from build123d import *

# Parameters (mm, degrees)
BOSS_EXTRUDE1_DEPTH = 20
SKETCH2_R           = 21
CUT_EXTRUDE1_DEPTH  = 21
SKETCH3_W           = 16
SKETCH3_H           = 76
BOSS_EXTRUDE2_DEPTH = 150


with BuildPart() as part:
    # Sketch1 → Boss-Extrude1 (new body)
    with BuildSketch(Plane.XY):
        with BuildLine():
            Line((0, 80), (0, 0))
            Line((0, 0), (60, 0))
            ThreePointArc((60, 0), (88.284271247, 11.715728753), (100, 40))
            ThreePointArc((100, 40), (88.284271247, 68.284271247), (60, 80))
            Line((60, 80), (0, 80))
        make_face()
    extrude(amount=BOSS_EXTRUDE1_DEPTH)

    # Sketch2 → Cut-Extrude1 (cut, through all)
    with BuildSketch(Plane.XY.offset(20)):
        with Locations((60, 40)):
            Circle(SKETCH2_R)
    extrude(amount=-CUT_EXTRUDE1_DEPTH, mode=Mode.SUBTRACT)

    # Sketch3 → Boss-Extrude2 (add)
    with BuildSketch(Plane.ZY):
        with Locations((10, 40)):
            Rectangle(SKETCH3_W, SKETCH3_H)
    extrude(amount=BOSS_EXTRUDE2_DEPTH)


solid = part.part
CAD build for the part. Positions are in the model's coordinates, mm. A direction names the side the tool comes from. Coordinates: 2 decimals unless noted, no trailing zeros. Order: outer loops, then holes, each group sorted by start corner. A loop starts at its lowest first (then second) coordinate and runs counter-clockwise, first axis right, second up. Notation, with made-up numbers: (29.25, -36) -> (86.25, -36) arc R18 cw to (86.25, -28) -> close; hole circle Ø1 at (-6.5, -12). An arc over 180 degrees is marked (long way). Answer in a Markdown table with one row per item.
1) Mould opens along Y. For faces 1 (the face through (38, 41, 0)), 2 (the face through (44.52, 54.19, 10.14)), 3 (the face through (-74, 2, 10)), 4 (the face through (-74, 78, 10)) say: pulls with the +Y half, pulls with the -Y half, needs draft (parallel to the pull), parting line crosses it, or undercut.
Check values:
| item | result |
|---|---|
| face 1 | needs draft |
| face 2 | undercut |
| face 3 | pulls with the -Y half |
| face 4 | pulls with the +Y half |
2) Which spindle directions (+Z, -Z, +X, -X, +Y, -Y) get a long thin tool onto all of the face, cutting with end or side? Do faces 5 (the face through (-150, 41, 10)), 6 (the face through (-74, 39, 2)), 7 (the face through (-74, 39, 18)). Say none if no direction does.
Check values:
| item | result |
|---|---|
| face 5 | +Z, -Z, -X, +Y, -Y |
| face 6 | -Z, -X, +Y, -Y |
| face 7 | +Z, -X, +Y, -Y |
3) Band-saw the part on D-D (x = -14.5). List the corners of the cut face in (y, z).
Check values:
| item | result |
|---|---|
| outline | (2, 2) -> (78, 2) -> (78, 18) -> (2, 18) -> close |
4) Band-saw the part on A-A (z = 5.5). List the corners of the cut face in (x, y), and give its area (3 significant figures).
Check values:
| item | result |
|---|---|
| outline | (-150, 2) -> (0, 2) -> (0, 0) -> (60, 0) arc R40 ccw to (60, 80) -> (0, 80) -> (0, 78) -> (-150, 78) -> close; hole circle Ø42 at (60, 40) |
| area | 17,300 mm2 |
5) Flat gauge pins, fed straight in: P1, Ø3, axis at x = -77.5, z = 6, coming from the +Y side; P2, Ø8, axis at y = 16, z = 7, coming from the +X side; P3, Ø23, axis at x = -92.5, y = 53, coming from the -Z side; P4, Ø1, axis at x = 64.5, y = 71, coming from the -Z side. Where does each tip first touch, or does it go through?
Check values:
| item | result |
|---|---|
| P1 | y = 78 |
| P2 | x = 94.64 |
| P3 | z = 2 |
| P4 | z = 0 |
6) Drill centre lines: line 1 (Y direction, x = 60, z = 9); line 2 (Z direction, x = -46.5, y = 9.5); line 3 (X direction, y = 58.5, z = 9.25). Where is each one in solid material? Low to high.
Check values:
| item | result |
|---|---|
| line 1 | 0 to 19, 61 to 80 |
| line 2 | 2 to 18 |
| line 3 | -150 to 50.06, 69.94 to 95.46 |
7) Band-saw the part on B-B (y = 49.5). List the corners of the cut face in (x, z), and give its area (3 significant figures).
Check values:
| item | result |
|---|---|
| outline | (-150, 2) -> (0, 2) -> (0, 0) -> (41.27, 0) -> (41.27, 20) -> (0, 20) -> (0, 18) -> (-150, 18) -> close; (78.73, 0) -> (98.86, 0) -> (98.86, 20) -> (78.73, 20) -> close |
| area | 3,630 mm2 |
8) Band-saw the part on C-C (y = 9.5). List the corners of the cut face in (x, z), and give its area (3 significant figures).
Check values:
| item | result |
|---|---|
| outline | (-150, 2) -> (0, 2) -> (0, 0) -> (85.88, 0) -> (85.88, 20) -> (0, 20) -> (0, 18) -> (-150, 18) -> close |
| area | 4,120 mm2 |
